```python
from build123d import *

# Parameters (mm, degrees)
SKETCH_219_R           = 1.55
EXTRUDE_1_DEPTH        = 2.75
SKETCH_940_W           = 10.000000002
SKETCH_940_H           = 4.75
EXTRUDE_2_DEPTH        = 2.75
SKETCH_1087_W          = 1
SKETCH_1087_H          = 6.95
EXTRUDE_1846_DEPTH     = 2.75
PCB_START              = -4
SKETCH_6_W             = 1
SKETCH_6_H             = 6.95
PCB_DEPTH              = 4
SKETCH_4_W             = 1.75
SKETCH_4_H             = 28.99988509
CUT_EXTRUDE_2332_DEPTH = 1.5
SKETCH_5_W             = 0.25
SKETCH_5_H             = 28.99988509
CUT_EXTRUDE_2_DEPTH    = 33.350081892
CHAMFER_1_SIZE         = 0.625
CUT_EXTRUDE_4_DEPTH    = 4


with BuildPart() as part:
    # Sketch 219 → 底座-1 (new body)
    with BuildSketch(Plane(origin=(0, 0, 0), x_dir=(1, 0, 0), z_dir=(0, 1, 0))):
        with BuildLine():
            Line((22.500000002, -14.24988509), (22.500000002, -7.263629174))
            Line((22.500000002, -7.263629174), (24.500000002, -7.263629174))
            Line((24.500000002, -7.263629174), (24.500000002, 0.312480077))
            Line((24.500000002, 0.312480077), (24.715186194, 2.08073674))
            ThreePointArc((24.715186194, 2.08073674), (20.15501929, 5.688743466), (16.252981126, 10))
            Line((16.252981126, 10), (12.5, 10))
            Line((12.5, 10), (12.5, -14.24988509))
            Line((12.5, -14.24988509), (22.500000002, -14.24988509))
        make_face()
        with Locations(Location((16.865979255, 0, 0), (0, 0, 270))):
            Circle(SKETCH_219_R, mode=Mode.SUBTRACT)
    extrude(amount=EXTRUDE_1_DEPTH)

    # Sketch 940 → 底座-2 (add)
    with BuildSketch(Plane(origin=(0, 0, 0), x_dir=(1, 0, 0), z_dir=(0, 1, 0))):
        with Locations((17.500000001, -16.62488509)):
            Rectangle(SKETCH_940_W, SKETCH_940_H)
    extrude(amount=EXTRUDE_2_DEPTH)

    # Sketch 1087 → Extrude 1846 (add)
    with BuildSketch(Plane(origin=(0, 0, 0), x_dir=(1, 0, 0), z_dir=(0, 1, 0))):
        with BuildLine():
            ThreePointArc((24.715186194, 2.08073674), (25.291636518, 1.705823535), (25.875319612, 1.342273079))
            Line((25.875319612, 1.342273079), (25.750000002, 0.312480077))
            Line((25.750000002, 0.312480077), (25.750000002, -14.213629174))
            Line((25.750000002, -14.213629174), (24.500000002, -14.213629174))
            Line((24.500000002, -14.213629174), (24.500000002, -7.263629174))
            Line((24.500000002, -7.263629174), (24.500000002, 0.312480077))
            Line((24.500000002, 0.312480077), (24.715186194, 2.08073674))
        make_face()
        with Locations((24.000000002, -10.738629174)):
            Rectangle(SKETCH_1087_W, SKETCH_1087_H)
        with Locations((23.000000002, -10.738629174)):
            Rectangle(SKETCH_1087_W, SKETCH_1087_H)
    extrude(amount=EXTRUDE_1846_DEPTH)

    # Sketch 6 → 底座卡榫-注意PCB突出部分 (add)
    with BuildSketch(Plane(origin=(0, 0, 0), x_dir=(1, 0, 0), z_dir=(0, 1, 0)).offset(PCB_START)):
        with Locations((24.000000002, -10.738629174)):
            Rectangle(SKETCH_6_W, SKETCH_6_H)
        with BuildLine():
            ThreePointArc((24.715186194, 2.08073674), (25.291636518, 1.705823535), (25.875319612, 1.342273079))
            Line((25.875319612, 1.342273079), (25.750000002, 0.312480077))
            Line((25.750000002, 0.312480077), (25.750000002, -14.213629174))
            Line((25.750000002, -14.213629174), (24.500000002, -14.213629174))
            Line((24.500000002, -14.213629174), (24.500000002, -7.263629174))
            Line((24.500000002, -7.263629174), (24.500000002, 0.312480077))
            Line((24.500000002, 0.312480077), (24.715186194, 2.08073674))
        make_face()
    extrude(amount=PCB_DEPTH)

    # 草图4 → Cut-Extrude 2332 (cut)
    with BuildSketch(Plane(origin=(0, 0, 0), x_dir=(1, 0, 0), z_dir=(0, 1, 0))):
        with Locations((13.375, -4.499942545)):
            Rectangle(SKETCH_4_W, SKETCH_4_H)
    extrude(amount=CUT_EXTRUDE_2332_DEPTH, mode=Mode.SUBTRACT)

    # 草图5 → 配合切除-2 (cut, through all)
    with BuildSketch(Plane(origin=(0, 0, 0), x_dir=(1, 0, 0), z_dir=(0, 1, 0))):
        with Locations((12.625, -4.499942545)):
            Rectangle(SKETCH_5_W, SKETCH_5_H)
    extrude(amount=CUT_EXTRUDE_2_DEPTH, mode=Mode.SUBTRACT)

    # 倒角1
    chamfer_1_edges = [part.edges().sort_by_distance(p)[0] for p in [
        (22.500000002, 1.375, 18.99988509),
        (22.500000002, 1.375, 14.213629174),
        (16.865979255, 2.75, -1.55),
        (20.661675073, 2.75, -5.223818951),
    ]]
    chamfer(chamfer_1_edges, length=CHAMFER_1_SIZE)

    # Sketch 6 2 → 切除-拉伸4 (cut)
    with BuildSketch(Plane.XZ.offset(4)):
        with BuildLine():
            Line((24.715186194, -2.08073674), (24.500000002, -0.312480077))
            Line((24.500000002, -0.312480077), (24.500000002, 7.263629174))
            Line((24.500000002, 7.263629174), (23.500000002, 7.263629174))
            Line((23.500000002, 7.263629174), (23.500000002, 7.513629174))
            Line((23.500000002, 7.513629174), (24.750000002, 7.513629174))
            Line((24.750000002, 7.513629174), (24.750000002, -0.312480077))
            Line((24.750000002, -0.312480077), (24.946632534, -1.928275128))
            ThreePointArc((24.946632534, -1.928275128), (24.830758909, -2.004277534), (24.715186194, -2.08073674))
        make_face()
    extrude(amount=-CUT_EXTRUDE_4_DEPTH, mode=Mode.SUBTRACT)


solid = part.part
```
The listing builds one solid part. Answer for the finished solid, in the listing's coordinates (mm). A direction names the side the tool comes from. Give positions to 0.01 mm unless a question says otherwise; leave off trailing zeros. Write each loop counter-clockwise with the first axis right and the second up, starting at its lowest first coordinate (ties: lowest second). Pieces come first, ordered by that corner, then holes. Notation, with made-up numbers: (79, 32.25) - (104, 32.25) arc R18 cw to (104, 38.25) - close; hole circle Ø4 at (-6.75, 36). An arc over 180 degrees is marked (long way). Use one line per item in the form item = value. Start each with the question number.
1) Find section B-B on z = 8. Determine the outline of the cut face in (x, y), plus the area to 3 significant figures.
2) A tool of negligible diameter and unlimited length cuts with its end or side. For faces 5 (the face through (22.5, 1, 17)), 6 (the face through (23.5, -2, 11)), 7 (the face through (24, -2, 7.514)), from which of +Z, -Z, +X, -X, +Y, -Y can it reach the whole face along a straight path? Write none if from no direction.
3) The mould has two halves that part along Z. Classify faces 1 (the face through (15, 2, -10)), 2 (the face through (24, -1, 14.214)), 3 (the face through (18.403, 1.048, -0.202)), 4 (the face through (12.75, 2, 5)): pulls with the +Z half, pulls with the -Z half, needs draft (parallel to the pull), parting line crosses it, or undercut.
4) Consider line 1 along Y through (x, z) = (15.25, 12); line 2 along X through (y, z) = (2.25, 10.5); line 3 along X through (y, z) = (0.4, 0). Determine where each line is inside the solid, lowest interval first. Write a range as from..to.
5) Find section C-C on y = -2.75. Determine the outline of the cut face in (x, z), plus the area to 3 significant figures.
6) Find section A-A on z = 0. Determine the outline of the cut face in (x, y) (3 decimals), plus the area to 3 significant figures.
7) Find section D-D on x = 13.75. Determine the outline of the cut face in (y, z), plus the area to 3 significant figures.
8) Flat-ended cylindrical pins translate along their axes: pin 1 Ø1 at (x, y) = (24, -3) entering from -Z; pin 2 Ø1.5 at (y, z) = (-1.5, 12) entering from -X; pin 3 Ø2 at (y, z) = (1.5, -3.5) entering from +X; pin 4 Ø1.5 at (x, y) = (16, -2) entering from -Z (3 decimals). Find the tip coordinate at first contact, or state that the pin passes through.
Geometry results:
q1.outline = (12.75, 1.5) - (14.25, 1.5) - (14.25, 0) - (23.5, 0) - (23.5, -4) - (25.75, -4) - (25.75, 2.75) - (12.75, 2.75) - close
q1.area = 42.5 mm2
q2.face_5 = +Z, +X, +Y, -Y
q2.face_6 = +Z, -Z, -X, -Y
q2.face_7 = -Z, -X, -Y
q3.face_1 = pulls with the -Z half
q3.face_2 = pulls with the +Z half
q3.face_3 = undercut
q3.face_4 = needs draft
q4.line_1 = 0..2.75
q4.line_2 = 12.75..25.75
q4.line_3 = 14.25..15.32, 18.42..25.75
q5.outline = (23.5, 7.51) - (24.75, 7.51) - (24.75, -0.31) - (24.95, -1.93) arc R35.11 cw to (25.88, -1.34) - (25.75, -0.31) - (25.75, 14.21) - (23.5, 14.21) - close
q5.area = 24.2 mm2
q6.outline = (12.75, 1.5) - (14.25, 1.5) - (14.25, 0) - (15.316, 0) - (15.316, 2.125) - (14.691, 2.75) - (12.75, 2.75) - close; (18.416, 0) - (24.75, 0) - (24.75, -4) - (25.75, -4) - (25.75, 2.75) - (19.041, 2.75) - (18.416, 2.125) - close
q6.area = 28.6 mm2
q7.outline = (1.5, -10) - (2.75, -10) - (2.75, 19) - (1.5, 19) - close
q7.area = 36.2 mm2
q8.pin_1 = 7.51
q8.pin_2 = 23.5
q8.pin_3 = 24.1
q8.pin_4 = through
